Source: CAD feature listing. Evaluate the final solid. Frame: model axes, mm. A direction names the side the tool comes from. Coordinates: 2 decimals unless noted, no trailing zeros. Write each loop counter-clockwise with the first axis right and the second up, starting at its lowest first coordinate (ties: lowest second). Pieces come first, ordered by that corner, then holes. Notation, with made-up numbers: M 46.25,31.25 L 76.25,31.25 A21 ccw 76.25,44.25 Z; hole C 45.25,79.25 d3. An arc over 180 degrees is marked long. Answer as CSV lines item,"result". Start each with the question number.
1. Section C-C on x = 2.75. Return the cut outline in (y, z).
2. Contact query for flat-ended pins moving along their axis: pin 1 Ø2 at (x, z) = (3.5, 5.5) entering from +Y; pin 2 Ø4 at (x, y) = (2.5, -1) entering from +Z; pin 3 Ø6 at (x, z) = (2, 16) entering from -Y. Output: stop coordinate, or through.
3. Line query: probe 1 along Y at (x, z) = (8.5, 14.75); probe 2 along Z at (x, y) = (2.75, -45.5); probe 3 along Y at (x, z) = (4, 20.5). Output: solid intervals per line, ascending. Write a range as [from, to].
4. Reachability of faces 1 (the face through (8, 1, 9)), 2 (the face through (2, 1, 9)), 3 (the face through (8, 9, 14)) from +Z, -Z, +X, -X, +Y, -Y: full face, straight path, thin tool, end or side. Return the list, or none.
```python
from build123d import *

# Parameters (mm, degrees)
F1_DEPTH = 10
F2_R     = 4.99999


# Not quite as in the source:
# - a fillet or chamfer is up to 0.001 mm smaller than in the source, because OpenCascade refuses the exact size


with BuildPart() as f1:
    # F0 (on Right) → F1 (new body)
    with BuildSketch(Plane.YZ):
        Polygon((0, 18.5156259346), (0, 0), (10, 0), (10, 28.5156259346), (-60, 28.5156259346), (-60, 18.5156259346), align=None)
    extrude(amount=F1_DEPTH)

    # F2 (radius 5 in the source; OpenCascade refuses exactly that, so slightly less here)
    f2_edges = [f1.edges().sort_by_distance(p)[0] for p in [
        (10, -30, 18.515626),
        (0, -30, 18.515626),
        (10, -25, 28.515626),
        (0, -25, 28.515626),
        (10, 0, 9.257813),
        (0, 0, 9.257813),
        (0, 10, 14.257813),
        (10, 10, 14.257813),
    ]]
    fillet(f2_edges, radius=F2_R)


solid = f1.part
```
Values:
1,outline,"M -60,19.05 L 0.53,19.05 L 0.53,0 L 9.47,0 L 9.47,27.98 L -60,27.98 Z"
2,pin 1,"y = 9.97"
2,pin 2,"z = 28.49"
2,pin 3,"y = 0"
3,probe 1,"[1.43, 8.57]"
3,probe 2,"[19.05, 27.98]"
3,probe 3,"[-60, 9.9]"
4,face 1,"-Z, +X, -Y"
4,face 2,"-Z, -X, -Y"
4,face 3,"+Z, -Z, +X, +Y"
